from build123d import *

# Parameters (mm, degrees)
F0_R     = 6.05
F1_DEPTH = 6
F2_R     = 21.5
F2_R_2   = 1.25
F3_DEPTH = 2


with BuildPart() as f1:
    # F0 (on Top) → F1 (new body)
    with BuildSketch(Plane.XY):
        Circle(F0_R)
        with BuildLine():
            Line((2.75, -1.3190905958), (-2.75, -1.3190905958))
            ThreePointArc((-2.75, -1.3190905958), (0, 3.05), (2.75, -1.3190905958))
        make_face(mode=Mode.SUBTRACT)
    extrude(amount=F1_DEPTH)

    # F2 (on face) → F3 (join)
    with BuildSketch(Plane.XY.offset(6)):
        Circle(F2_R)
        with BuildLine():
            ThreePointArc((12.2499946096, 13.8631753962), (16.02146997, 9.25), (18.130859375, 3.67721883))
            ThreePointArc((18.130859375, 3.67721883), (19.6822990335, 2.1220682902), (20.25, 0))
            ThreePointArc((20.25, 0), (19.6822990335, -2.1220682902), (18.130859375, -3.67721883))
            ThreePointArc((18.130859375, -3.67721883), (16.02146997, -9.25), (12.2499946096, -13.8631753962))
            ThreePointArc((12.2499946096, -13.8631753962), (10.125, -17.5370144266), (5.8808647654, -17.5403942262))
            ThreePointArc((5.8808647654, -17.5403942262), (0, -18.5), (-5.8808647654, -17.5403942262))
            ThreePointArc((-5.8808647654, -17.5403942262), (-10.125, -17.5370144266), (-12.2499946096, -13.8631753962))
            ThreePointArc((-12.2499946096, -13.8631753962), (-16.02146997, -9.25), (-18.130859375, -3.67721883))
            ThreePointArc((-18.130859375, -3.67721883), (-20.25, 0), (-18.130859375, 3.67721883))
            ThreePointArc((-18.130859375, 3.67721883), (-16.02146997, 9.25), (-12.2499946096, 13.8631753962))
            ThreePointArc((-12.2499946096, 13.8631753962), (-10.125, 17.5370144266), (-5.8808647654, 17.5403942262))
            ThreePointArc((-5.8808647654, 17.5403942262), (0, 18.5), (5.8808647654, 17.5403942262))
            ThreePointArc((5.8808647654, 17.5403942262), (10.125, 17.5370144266), (12.2499946096, 13.8631753962))
        make_face(mode=Mode.SUBTRACT)
        with BuildLine():
            ThreePointArc((-12.0235065699, 1.5), (-14.5728834228, 4.0032284815), (-18.130859375, 3.67721883))
            ThreePointArc((-18.130859375, 3.67721883), (-18.5, 0), (-18.130859375, -3.67721883))
            ThreePointArc((-18.130859375, -3.67721883), (-14.5728834228, -4.0032284815), (-12.0235065699, -1.5))
            Line((-12.0235065699, -1.5), (-14, -1.5))
            Line((-14, -1.5), (-14, 1.5))
            Line((-14, 1.5), (-12.0235065699, 1.5))
        make_face()
        with Locations((-16, 0)):
            Circle(F2_R_2, mode=Mode.SUBTRACT)
        with BuildLine():
            ThreePointArc((-3.75, 13.8564064606), (-4.3210854354, 15.9843368228), (-5.8808647654, 17.5403942262))
            ThreePointArc((-5.8808647654, 17.5403942262), (-9.25, 16.02146997), (-12.2499946096, 13.8631753962))
            ThreePointArc((-12.2499946096, 13.8631753962), (-10.7533392736, 10.6188730098), (-7.3107913906, 9.6626621321))
            Line((-7.3107913906, 9.6626621321), (-8.2990381057, 11.374355653))
            Line((-8.2990381057, 11.374355653), (-5.7009618943, 12.874355653))
            Line((-5.7009618943, 12.874355653), (-4.7127151792, 11.1626621321))
            ThreePointArc((-4.7127151792, 11.1626621321), (-3.9979092659, 12.4261023824), (-3.75, 13.8564064606))
        make_face()
        with Locations((-8, 13.8564064606)):
            Circle(F2_R_2, mode=Mode.SUBTRACT)
        with BuildLine():
            ThreePointArc((12.25, 13.8564064606), (12.2499986524, 13.8597909294), (12.2499946096, 13.8631753962))
            ThreePointArc((12.2499946096, 13.8631753962), (9.25, 16.02146997), (5.8808647654, 17.5403942262))
            ThreePointArc((5.8808647654, 17.5403942262), (3.8195441493, 14.6221014913), (4.7127151792, 11.1626621321))
            Line((4.7127151792, 11.1626621321), (5.7009618943, 12.874355653))
            Line((5.7009618943, 12.874355653), (8.2990381057, 11.374355653))
            Line((8.2990381057, 11.374355653), (7.3107913906, 9.6626621321))
            ThreePointArc((7.3107913906, 9.6626621321), (10.7507602049, 10.6166814267), (12.25, 13.8564064606))
        make_face()
        with Locations((8, 13.8564064606)):
            Circle(F2_R_2, mode=Mode.SUBTRACT)
        with BuildLine():
            ThreePointArc((18.130859375, -3.67721883), (18.4074835113, -1.8478503135), (18.5, 0))
            ThreePointArc((18.5, 0), (18.4074835113, 1.8478503135), (18.130859375, 3.67721883))
            ThreePointArc((18.130859375, 3.67721883), (14.5728834228, 4.0032284815), (12.0235065699, 1.5))
            Line((12.0235065699, 1.5), (14, 1.5))
            Line((14, 1.5), (14, -1.5))
            Line((14, -1.5), (12.0235065699, -1.5))
            ThreePointArc((12.0235065699, -1.5), (14.5728834228, -4.0032284815), (18.130859375, -3.67721883))
        make_face()
        with Locations((16, 0)):
            Circle(F2_R_2, mode=Mode.SUBTRACT)
        with BuildLine():
            ThreePointArc((5.8808647654, -17.5403942262), (9.25, -16.02146997), (12.2499946096, -13.8631753962))
            ThreePointArc((12.2499946096, -13.8631753962), (12.2499986524, -13.8597909294), (12.25, -13.8564064606))
            ThreePointArc((12.25, -13.8564064606), (10.7507602049, -10.6166814267), (7.3107913906, -9.6626621321))
            Line((7.3107913906, -9.6626621321), (8.2990381057, -11.374355653))
            Line((8.2990381057, -11.374355653), (5.7009618943, -12.874355653))
            Line((5.7009618943, -12.874355653), (4.7127151792, -11.1626621321))
            ThreePointArc((4.7127151792, -11.1626621321), (3.8195441493, -14.6221014913), (5.8808647654, -17.5403942262))
        make_face()
        with Locations((8, -13.8564064606)):
            Circle(F2_R_2, mode=Mode.SUBTRACT)
        with BuildLine():
            ThreePointArc((-12.2499946096, -13.8631753962), (-9.25, -16.02146997), (-5.8808647654, -17.5403942262))
            ThreePointArc((-5.8808647654, -17.5403942262), (-4.3210854354, -15.9843368228), (-3.75, -13.8564064606))
            ThreePointArc((-3.75, -13.8564064606), (-3.9979092659, -12.4261023824), (-4.7127151792, -11.1626621321))
            Line((-4.7127151792, -11.1626621321), (-5.7009618943, -12.874355653))
            Line((-5.7009618943, -12.874355653), (-8.2990381057, -11.374355653))
            Line((-8.2990381057, -11.374355653), (-7.3107913906, -9.6626621321))
            ThreePointArc((-7.3107913906, -9.6626621321), (-10.7533392736, -10.6188730098), (-12.2499946096, -13.8631753962))
        make_face()
        with Locations((-8, -13.8564064606)):
            Circle(F2_R_2, mode=Mode.SUBTRACT)
        with BuildLine():
            ThreePointArc((-12.2499946096, 13.8631753962), (-9.25, 16.02146997), (-5.8808647654, 17.5403942262))
            ThreePointArc((-5.8808647654, 17.5403942262), (-10.125, 17.5370144266), (-12.2499946096, 13.8631753962))
        make_face()
        with BuildLine():
            ThreePointArc((-18.130859375, -3.67721883), (-18.5, 0), (-18.130859375, 3.67721883))
            ThreePointArc((-18.130859375, 3.67721883), (-20.25, 0), (-18.130859375, -3.67721883))
        make_face()
        with BuildLine():
            ThreePointArc((-12.2499946096, -13.8631753962), (-10.125, -17.5370144266), (-5.8808647654, -17.5403942262))
            ThreePointArc((-5.8808647654, -17.5403942262), (-9.25, -16.02146997), (-12.2499946096, -13.8631753962))
        make_face()
        with BuildLine():
            ThreePointArc((5.8808647654, -17.5403942262), (10.125, -17.5370144266), (12.2499946096, -13.8631753962))
            ThreePointArc((12.2499946096, -13.8631753962), (9.25, -16.02146997), (5.8808647654, -17.5403942262))
        make_face()
        with BuildLine():
            ThreePointArc((18.130859375, 3.67721883), (18.4074835113, 1.8478503135), (18.5, 0))
            ThreePointArc((18.5, 0), (18.4074835113, -1.8478503135), (18.130859375, -3.67721883))
            ThreePointArc((18.130859375, -3.67721883), (19.6822990335, -2.1220682902), (20.25, 0))
            ThreePointArc((20.25, 0), (19.6822990335, 2.1220682902), (18.130859375, 3.67721883))
        make_face()
        with BuildLine():
            ThreePointArc((5.8808647654, 17.5403942262), (9.25, 16.02146997), (12.2499946096, 13.8631753962))
            ThreePointArc((12.2499946096, 13.8631753962), (10.125, 17.5370144266), (5.8808647654, 17.5403942262))
        make_face()
        with BuildLine():
            ThreePointArc((-4.7127151792, 11.1626621321), (-5.875, 10.1757984945), (-7.3107913906, 9.6626621321))
            Line((-7.3107913906, 9.6626621321), (-4.2295883953, 4.3258619958))
            ThreePointArc((-4.2295883953, 4.3258619958), (-3.025, 5.2394536929), (-1.6315121839, 5.8258619958))
            Line((-1.6315121839, 5.8258619958), (-4.7127151792, 11.1626621321))
        make_face()
        with BuildLine():
            Line((-8.2990381057, 11.374355653), (-7.3107913906, 9.6626621321))
            ThreePointArc((-7.3107913906, 9.6626621321), (-5.875, 10.1757984945), (-4.7127151792, 11.1626621321))
            Line((-4.7127151792, 11.1626621321), (-5.7009618943, 12.874355653))
            Line((-5.7009618943, 12.874355653), (-8.2990381057, 11.374355653))
        make_face()
        with BuildLine():
            Line((5.7009618943, 12.874355653), (4.7127151792, 11.1626621321))
            ThreePointArc((4.7127151792, 11.1626621321), (5.875, 10.1757984945), (7.3107913906, 9.6626621321))
            Line((7.3107913906, 9.6626621321), (8.2990381057, 11.374355653))
            Line((8.2990381057, 11.374355653), (5.7009618943, 12.874355653))
        make_face()
        with BuildLine():
            ThreePointArc((7.3107913906, 9.6626621321), (5.875, 10.1757984945), (4.7127151792, 11.1626621321))
            Line((4.7127151792, 11.1626621321), (1.6315121839, 5.8258619958))
            ThreePointArc((1.6315121839, 5.8258619958), (3.025, 5.2394536929), (4.2295883953, 4.3258619958))
            Line((4.2295883953, 4.3258619958), (7.3107913906, 9.6626621321))
        make_face()
        with BuildLine():
            ThreePointArc((12.0235065699, -1.5), (11.75, 0), (12.0235065699, 1.5))
            Line((12.0235065699, 1.5), (5.8611005792, 1.5))
            ThreePointArc((5.8611005792, 1.5), (6.0025893789, 0.7559237712), (6.05, 0))
            ThreePointArc((6.05, 0), (6.0025893789, -0.7559237712), (5.8611005792, -1.5))
            Line((5.8611005792, -1.5), (12.0235065699, -1.5))
        make_face()
        with BuildLine():
            Line((14, 1.5), (12.0235065699, 1.5))
            ThreePointArc((12.0235065699, 1.5), (11.75, 0), (12.0235065699, -1.5))
            Line((12.0235065699, -1.5), (14, -1.5))
            Line((14, -1.5), (14, 1.5))
        make_face()
        with BuildLine():
            Line((1.6315121839, -5.8258619958), (4.7127151792, -11.1626621321))
            ThreePointArc((4.7127151792, -11.1626621321), (5.875, -10.1757984945), (7.3107913906, -9.6626621321))
            Line((7.3107913906, -9.6626621321), (4.2295883953, -4.3258619958))
            ThreePointArc((4.2295883953, -4.3258619958), (3.025, -5.2394536929), (1.6315121839, -5.8258619958))
        make_face()
        with BuildLine():
            ThreePointArc((7.3107913906, -9.6626621321), (5.875, -10.1757984945), (4.7127151792, -11.1626621321))
            Line((4.7127151792, -11.1626621321), (5.7009618943, -12.874355653))
            Line((5.7009618943, -12.874355653), (8.2990381057, -11.374355653))
            Line((8.2990381057, -11.374355653), (7.3107913906, -9.6626621321))
        make_face()
        with BuildLine():
            Line((-4.2295883953, -4.3258619958), (-7.3107913906, -9.6626621321))
            ThreePointArc((-7.3107913906, -9.6626621321), (-5.875, -10.1757984945), (-4.7127151792, -11.1626621321))
            Line((-4.7127151792, -11.1626621321), (-1.6315121839, -5.8258619958))
            ThreePointArc((-1.6315121839, -5.8258619958), (-3.025, -5.2394536929), (-4.2295883953, -4.3258619958))
        make_face()
        with BuildLine():
            ThreePointArc((-4.7127151792, -11.1626621321), (-5.875, -10.1757984945), (-7.3107913906, -9.6626621321))
            Line((-7.3107913906, -9.6626621321), (-8.2990381057, -11.374355653))
            Line((-8.2990381057, -11.374355653), (-5.7009618943, -12.874355653))
            Line((-5.7009618943, -12.874355653), (-4.7127151792, -11.1626621321))
        make_face()
        with BuildLine():
            Line((-5.8611005792, 1.5), (-12.0235065699, 1.5))
            ThreePointArc((-12.0235065699, 1.5), (-11.8189357169, 0.7623657003), (-11.75, 0))
            ThreePointArc((-11.75, 0), (-11.8189357169, -0.7623657003), (-12.0235065699, -1.5))
            Line((-12.0235065699, -1.5), (-5.8611005792, -1.5))
            ThreePointArc((-5.8611005792, -1.5), (-6.05, 0), (-5.8611005792, 1.5))
        make_face()
        with BuildLine():
            ThreePointArc((-11.75, 0), (-11.8189357169, 0.7623657003), (-12.0235065699, 1.5))
            Line((-12.0235065699, 1.5), (-14, 1.5))
            Line((-14, 1.5), (-14, -1.5))
            Line((-14, -1.5), (-12.0235065699, -1.5))
            ThreePointArc((-12.0235065699, -1.5), (-11.8189357169, -0.7623657003), (-11.75, 0))
        make_face()
    extrude(amount=-F3_DEPTH)


solid = f1.part
Input: part model. Units: mm. Frame: model coordinates. A direction names the side the tool comes from. Give positions to 0.01 mm unless a question says otherwise; leave off trailing zeros. Order: outer loops, then holes, each group sorted by start corner. A loop starts at its lowest first (then second) coordinate and runs counter-clockwise, first axis right, second up. Notation, with made-up numbers: (36, 22.5) - (78, 22.5) arc R23 ccw to (78, 56.5) - close; hole circle Ø8 at (8.5, -15). An arc over 180 degrees is marked (long way). Answer as a JSON object with one key per item and string values. Group by question number.
Q1. Set-up query: faces 1 (the face through (-3.194, -8.532, 5.014)), 2 (the face through (4, 0, 6)). Return all of +Z, -Z, +X, -X, +Y, -Y with unobstructed straight access to the full face (end or side cutting, diameter ignored); none if empty.
Q2. Cut plane D-D, the plane z = 0.95. Output: boundary loops of the cut face in (x, y).
Q3. Cut plane A-A, the plane x = 0. Output: boundary loops of the cut face in (y, z), then the cut area to 3 significant figures.
Q4. Line query: probe 1 along X at (y, z) = (9, 4.7); probe 2 along X at (y, z) = (8, 5.7); probe 3 along Y at (x, z) = (8, 4.6). Output: solid intervals per line, ascending.
Q5. Cut plane C-C, the plane x = 8. Output: boundary loops of the cut face in (y, z), then the cut area to 3 significant figures.
Q6. Cut plane B-B, the plane y = 0. Output: boundary loops of the cut face in (x, z), then the cut area to 3 significant figures.
Q7. Mould query, pull axis Y, two halves, no side actions, for faces 3 (the face through (-2.799, 21.317, 5.014)), 4 (the face through (-8.163, 15.096, 5.014)), 5 (the face through (4, 5, 4)). Classes: pulls with the +Y half, pulls with the -Y half, needs draft (parallel to the pull), parting line crosses it, or undercut.
Q8. First-contact query: pin 1 Ø2 at (x, z) = (-8.5, 4.5) entering from -Y; pin 2 Ø8 at (x, y) = (-13.5, -12.5) entering from +Z; pin 3 Ø3 at (x, y) = (-8, -13.86) entering from -Z; pin 4 Ø0.6 at (x, z) = (9, 5) entering from -Y. Flat tips, straight axial feed; report the tip coordinate or a pass-through.
Results:
{
 "1": {"face 1": "+Z, -Z", "face 2": "+Z, +X, -X, +Y, -Y"},
 "2": {"outline": "circle Ø12.1 at (0, 0); hole (-2.75, -1.32) - (2.75, -1.32) arc R3.05 ccw (long way) to start"},
 "3": {"outline": "(-21.5, 4) - (-18.5, 4) - (-18.5, 6) - (-21.5, 6) - close; (-6.05, 0) - (-1.32, 0) - (-1.32, 6) - (-6.05, 6) - close; (3.05, 0) - (6.05, 0) - (6.05, 6) - (3.05, 6) - close; (18.5, 4) - (21.5, 4) - (21.5, 6) - (18.5, 6) - close", "area": "58.4 mm^2"},
 "4": {"probe 1": "-19.53 to -16.16, -6.93 to -3.46, 3.46 to 6.93, 16.16 to 19.53", "probe 2": "-19.96 to -16.68, -6.35 to -2.89, 2.89 to 6.35, 16.68 to 19.96", "probe 3": "-19.96 to -15.11, -12.61 to -9.61, -1.5 to 1.5, 9.61 to 12.61, 15.11 to 19.96"},
 "5": {"outline": "(-19.96, 4) - (-15.11, 4) - (-15.11, 6) - (-19.96, 6) - close; (-12.61, 4) - (-9.61, 4) - (-9.61, 6) - (-12.61, 6) - close; (-1.5, 4) - (1.5, 4) - (1.5, 6) - (-1.5, 6) - close; (9.61, 4) - (12.61, 4) - (12.61, 6) - (9.61, 6) - close; (15.11, 4) - (19.96, 4) - (19.96, 6) - (15.11, 6) - close", "area": "37.4 mm^2"},
 "6": {"outline": "(-21.5, 4) - (-17.25, 4) - (-17.25, 6) - (-21.5, 6) - close; (-14.75, 4) - (-6.05, 4) - (-6.05, 0) - (-3.05, 0) - (-3.05, 6) - (-14.75, 6) - close; (3.05, 0) - (6.05, 0) - (6.05, 4) - (14.75, 4) - (14.75, 6) - (3.05, 6) - close; (17.25, 4) - (21.5, 4) - (21.5, 6) - (17.25, 6) - close", "area": "87.8 mm^2"},
 "7": {"face 3": "parting line crosses it", "face 4": "undercut", "face 5": "needs draft"},
 "8": {"pin 1": "y = -20.15", "pin 2": "z = 6", "pin 3": "z = 4", "pin 4": "y = -19.66"}
}
